Can you work these out from the model? Positions are in its coordinate system, mm. Face numbers are marked on the shaded views. A direction names the side the tool comes from. Give positions to 0.01 mm unless a question says otherwise; leave off trailing zeros. Order: outer loops, then holes, each group sorted by start corner. A loop starts at its lowest first (then second) coordinate and runs counter-clockwise, first axis right, second up.
Item 1: If I drill on line 1 along X through (y, z) = (0.75, 4.75); line 2 along Z through (x, y) = (18, -3.75); line 3 along X through (y, z) = (-4, 9.5), over which ranges is the centre line in solid material (lowest first)?
Item 2: I want a section at A-A, the plane y = 0. Write out the boundary of the cut face in (x, z), then the cut area to 3 significant figures.
Item 3: I'm going to push flat-ended pins straight in: pin 1 Ø1 at (y, z) = (-7, 9) entering from -X; pin 2 Ø9 at (x, y) = (0, 0) entering from -Z; pin 3 Ø3 at (x, z) = (9, 7.5) entering from -Y; pin 4 Ø5.5 at (x, y) = (-12, 4.5) entering from +Z. Where does each tip first touch, or does it pass through?
Item 4: If we mould it in two halves opening along Y, with no side actions, what happens to the marked faces 1, 2, 3 and 4? For each: +Y half, -Y half, draft (parallel to the pull), parting line (faces both ways), or undercut.
Item 5: I want a section at D-D, the plane y = -10.75. Write out the boundary of the cut face in (x, z).
Item 6: Which directions (+Z, -Z, +X, -X, +Y, -Y) give clear straight access to the entire face, cutting with the end or side of a thin tool? Please do the marked faces 5, 6 and 7.
Item 7: I want a section at B-B, the plane x = -16.5. Write out the boundary of the cut face in (y, z), then the cut area to 3 significant figures.
Item 8: I want a section at C-C, the plane z = 6.25. Write out the boundary of the cut face in (x, y), then the cut area to 3 significant figures.
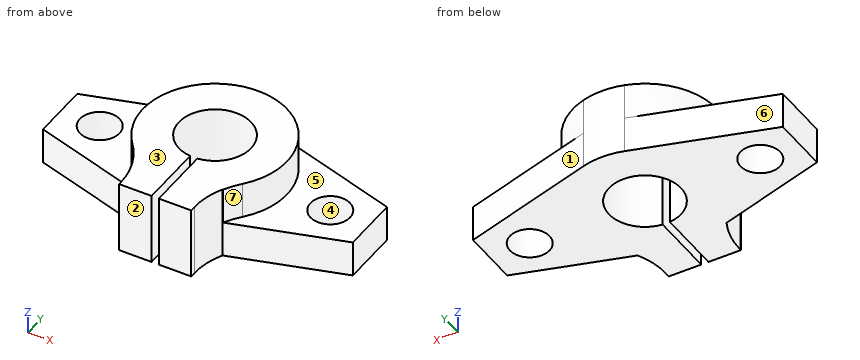
```python
from build123d import *

# Parameters (mm, degrees)
SKETCH_1_R               = 2.75
EXTRUDE_4_DEPTH          = 5
EXTRUDE_5_DEPTH          = 5
EXTRUDE_START            = -10
SKETCH_6_R               = 5.188573112
EXTRUDE_6_DEPTH          = 10
CUT_EXTRUDE_1_DEPTH      = 28.536339626
CUT_EXTRUDE_1_DEPTH_BACK = 28.536339626


with BuildPart() as part:
    # Эскиз1 → Бобышка-Вытянуть4 (new body)
    with BuildSketch(Plane.XY):
        with BuildLine():
            Line((-21.5, 4), (-21.5, -4))
            Line((-21.5, -4), (-6.226230763, -8.574183073))
            ThreePointArc((-6.226230763, -8.574183073), (-5.310888369, -11.044106025), (-5, -13.659774106))
            Line((-5, -13.659774106), (-5, -14))
            Line((-5, -14), (-0.5, -14))
            Line((-0.5, -14), (-0.5, -5.164425519))
            ThreePointArc((-0.5, -5.164425519), (0, 5.188573112), (0.5, -5.164425519))
            Line((0.5, -5.164425519), (0.5, -14))
            Line((0.5, -14), (5, -14))
            Line((5, -14), (5, -13.228756555))
            ThreePointArc((5, -13.228756555), (5.287888706, -10.846552908), (6.134978844, -8.601511166))
            Line((6.134978844, -8.601511166), (21.5, -4))
            Line((21.5, -4), (21.5, 4))
            Line((21.5, 4), (2.868905356, 9.579633712))
            ThreePointArc((2.868905356, 9.579633712), (0, 10), (-2.868905356, 9.579633712))
            Line((-2.868905356, 9.579633712), (-21.5, 4))
        make_face()
        with Locations((-16, 0)):
            Circle(SKETCH_1_R, mode=Mode.SUBTRACT)
        with Locations((16, 0)):
            Circle(SKETCH_1_R, mode=Mode.SUBTRACT)
    extrude(amount=EXTRUDE_4_DEPTH)

    # Эскиз5 → Бобышка-Вытянуть5 (add)
    with BuildSketch(Plane.XY.offset(5)):
        with BuildLine():
            Line((-5, -14), (-0.5, -14))
            Line((-0.5, -14), (-0.5, -5.164425519))
            ThreePointArc((-0.5, -5.164425519), (-3.48762128, 3.841586749), (5.188573112, 0))
            ThreePointArc((5.188573112, 0), (3.841586749, -3.48762128), (0.5, -5.164425519))
            Line((0.5, -5.164425519), (0.5, -14))
            Line((0.5, -14), (5, -14))
            Line((5, -14), (5, -13.659774106))
            Line((5, -13.659774106), (5, -13.228756555))
            ThreePointArc((5, -13.228756555), (5.287888706, -10.846552908), (6.134978844, -8.601511166))
            Line((6.134978844, -8.601511166), (6.226230763, -8.574183073))
            ThreePointArc((6.226230763, -8.574183073), (6.870989069, -7.474637071), (7.636932983, -6.455792331))
            ThreePointArc((7.636932983, -6.455792331), (9.585242923, 2.850108438), (2.868905356, 9.579633712))
            ThreePointArc((2.868905356, 9.579633712), (0, 10), (-2.868905356, 9.579633712))
            ThreePointArc((-2.868905356, 9.579633712), (-9.585242923, 2.850108438), (-7.636932983, -6.455792331))
            ThreePointArc((-7.636932983, -6.455792331), (-6.870989069, -7.474637071), (-6.226230763, -8.574183073))
            ThreePointArc((-6.226230763, -8.574183073), (-5.310888369, -11.044106025), (-5, -13.659774106))
            Line((-5, -13.659774106), (-5, -14))
        make_face()
    extrude(amount=EXTRUDE_5_DEPTH)

    # Эскиз6 → Бобышка-Вытянуть6 (add)
    with BuildSketch(Plane.XY.offset(10).offset(EXTRUDE_START)):
        Circle(SKETCH_6_R)
    extrude(amount=EXTRUDE_6_DEPTH)

    # Эскиз7 → Вырез-Вытянуть1 (cut, two sides: drawn at the far end of the back side and taken through both)
    with BuildSketch(Plane.XY.offset(10).offset(-CUT_EXTRUDE_1_DEPTH_BACK)):
        with BuildLine():
            Line((-0.5, -4.974937186), (-0.5, -5.164425519))
            ThreePointArc((-0.5, -5.164425519), (0, -5.188573112), (0.5, -5.164425519))
            Line((0.5, -5.164425519), (0.5, -4.974937186))
            ThreePointArc((0.5, -4.974937186), (0, 5), (-0.5, -4.974937186))
        make_face()
    extrude(amount=CUT_EXTRUDE_1_DEPTH + CUT_EXTRUDE_1_DEPTH_BACK, mode=Mode.SUBTRACT)


solid = part.part
```
Results list:
1. line 1: x = -21.5 to -18.65, -13.35 to -4.94, 4.94 to 13.35, 18.65 to 21.5
1. line 2: z = 0 to 5
1. line 3: x = -9.17 to -3, 3 to 9.17
2. outline: (-21.5, 0) - (-18.75, 0) - (-18.75, 5) - (-21.5, 5) - close; (-13.25, 0) - (-5, 0) - (-5, 10) - (-10, 10) - (-10, 5) - (-13.25, 5) - close; (5, 0) - (13.25, 0) - (13.25, 5) - (10, 5) - (10, 10) - (5, 10) - close; (18.75, 0) - (21.5, 0) - (21.5, 5) - (18.75, 5) - close
2. area: 160 mm2
3. pin 1: stops at x = -7.6
3. pin 2: passes through
3. pin 3: stops at y = -6.62
3. pin 4: stops at z = 5
4. face 1: +Y half
4. face 2: -Y half
4. face 3: draft
4. face 4: undercut
5. outline: (-5.39, 0) - (-0.5, 0) - (-0.5, 10) - (-5.39, 10) - close; (0.5, 0) - (5.31, 0) - (5.31, 10) - (0.5, 10) - close
6. face 5: +Z, +X
6. face 6: +Z, -Z, -X, +Y
6. face 7: +Z, +X, -Y
7. outline: (-5.5, 0) - (-2.7, 0) - (-2.7, 5) - (-5.5, 5) - close; (2.7, 0) - (5.5, 0) - (5.5, 5) - (2.7, 5) - close
7. area: 27.9 mm2
8. outline: (-7.64, -6.46) arc R11.16 cw to (-5, -13.66) - (-5, -14) - (-0.5, -14) - (-0.5, -4.97) arc R5 cw (long way) to (0.5, -4.97) - (0.5, -14) - (5, -14) - (5, -13.23) arc R10 cw to (6.13, -8.6) - (6.23, -8.57) arc R11.16 cw to (7.64, -6.46) arc R10 ccw (long way) to start
8. area: 276 mm2
